Study the drawing (mm; zero at the part's minimum x, y, z) and answer. Round coordinates to 2 decimals unless told otherwise and drop trailing zeros. Write each loop counter-clockwise with the first axis right and the second up, starting at its lowest first coordinate (ties: lowest second). Pieces come first, ordered by that corner, then holes.
(1) Find the intervals of material crossed by probe 1 along X at (y, z) = (3.9, 10); probe 2 along Z at (x, y) = (55, 3.1), in increasing order.
(2) A cutting plane is placed at D-D, the plane x = 41.5. Give the vertices of the cut face in (y, z).
(3) A cutting plane is placed at B-B, the plane y = 35. Give the vertices of the cut face in (x, z).
(4) Each of these flat-tipped pins is pushed along its axis until it touches: pin 1 Ø5 at (y, z) = (21.5, 10) entering from +X; pin 2 Ø4 at (y, z) = (44, 11.5) entering from -X; pin 3 Ø5 at (x, z) = (55, 10) entering from -Y; pin 4 Ø4 at (y, z) = (35, 4) entering from +X. Where does it stop, or does it pass through?
(5) A cutting plane is placed at A-A, the plane x = 15. Give the vertices of the cut face in (y, z), and give its area (3 significant figures).
(6) A cutting plane is placed at C-C, the plane z = 10. Give the number of separate pieces and of enclosed holes in the cut face, and give its area (3 significant figures).
(7) The mould has two halves that part along Z. Classify the marked faces 1, 2 and 3: +Z half, -Z half, draft (parallel to the pull), parting line (faces both ways), or undercut.
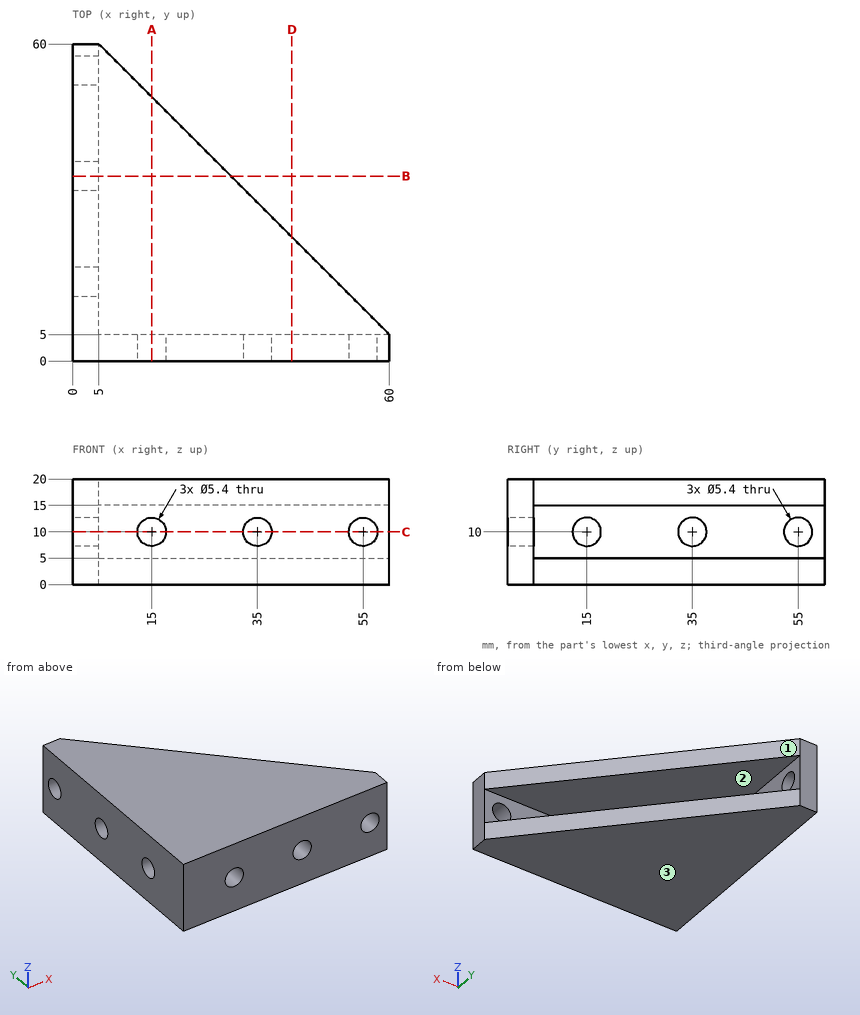
Solutions:
1. probe 1: x = 0 to 12.3, 17.7 to 32.3, 37.7 to 52.3, 57.7 to 60
1. probe 2: z = 0 to 7.3, 12.7 to 20
2. outline: (0, 0) - (23.5, 0) - (23.5, 5) - (5, 5) - (5, 15) - (23.5, 15) - (23.5, 20) - (0, 20) - close
3. outline: (0, 0) - (30, 0) - (30, 5) - (5, 5) - (5, 7.3) - (0, 7.3) - close; (0, 12.7) - (5, 12.7) - (5, 15) - (30, 15) - (30, 20) - (0, 20) - close
4. pin 1: stops at x = 5
4. pin 2: stops at x = 0
4. pin 3: passes through
4. pin 4: stops at x = 32
5. outline: (0, 0) - (50, 0) - (50, 5) - (5, 5) - (5, 7.3) - (0, 7.3) - close; (0, 12.7) - (5, 12.7) - (5, 15) - (50, 15) - (50, 20) - (0, 20) - close
5. area: 523 mm2
6. separate pieces: 7
6. enclosed holes: 0
6. area: 413 mm2
7. face 1: draft
7. face 2: undercut
7. face 3: -Z half
